For this review, take the finished solid that the model builds, in its own axes (mm). A direction names the side the tool comes from. Give positions to 0.01 mm unless a question says otherwise; leave off trailing zeros. Write each loop counter-clockwise with the first axis right and the second up, starting at its lowest first coordinate (ties: lowest second). Pieces come first, ordered by that corner, then holes.
1) For P1, Ø4, axis at x = -2, z = 25.5, coming from the -Y side; P2, Ø11, axis at y = -11, z = 47, coming from the -X side; P3, Ø3, axis at x = -0.5, y = 4.5, coming from the -Z side; P4, Ø3, axis at x = 0.5, z = 27.5, coming from the +Y side, all flat-tipped, find the tip position at first contact; note any pin that passes through.
2) Wall thickness on line 1 along Z through (x, y) = (-1.5, -16.5); line 2 along Y through (x, z) = (4, -2.5); line 3 along Y through (x, z) = (-0.75, 39): over which ranges is each line inside the solid? List them lowest first.
3) We need section C-C on x = 4. Give the boundary of the cut face in (y, z).
4) Draft analysis for pull direction Z (two halves, no side actions). For faces 4 (the face through (2, 15.24, 2)), 5 (the face through (2.451, 2.348, 10.305)), 6 (the face through (0.022, -0.354, 42.917)), 7 (the face through (0.54, 7.73, -2.44)), state which applies: pulls with the +Z half, pulls with the -Z half, needs draft (parallel to the pull), parting line crosses it, or undercut.
5) Machinability: for faces 1 (the face through (0, -17, 71.438)), 2 (the face through (-1.588, -1.5, 47.5)), 3 (the face through (0.07, 8.91, 8.89)), which of the approach directions +Z, -Z, +X, -X, +Y, -Y give a long, thin tool a straight path to every point of the face, cutting with its end or side? Answer none if there is none.
6) We need section D-D on z = 69. Give the boundary of the cut face in (x, y).
7) We need section A-A on z = 0. Give the boundary of the cut face in (x, y), and give its area (3 significant figures).
from build123d import *

# Parameters (mm, degrees)
F2_DEPTH      = 1.5875
F2_DEPTH_BACK = 1.5875
F3_DEPTH      = 9.525
F3_DEPTH_BACK = 9.525
F4_T1_DEPTH   = 62.865
F4_T6_DEPTH   = 62.865
F4_T11_DEPTH  = 62.865
F4_T16_DEPTH  = 62.865
F4_T21_DEPTH  = 62.865
F5_R          = 2.5
F6_DEPTH      = 34.1227081721
F7_R          = 1.3462
F8_DEPTH      = 25.4
F9_R          = 7.62
F10_R         = 0.635
F11_DEPTH     = 25.4
F12_R         = 1.27
F14_DEPTH     = 34.1227081721


# Not quite as in the source:
# - a fillet or chamfer that OpenCascade refuses, or shapes differently, is made with other operations: its cross-section is extruded or revolved along the edge and cut away or added
# - a feature names something its author has since deleted; it is built from what else it names


with BuildPart() as f2:
    # F1 (on Right) → F2 (new body, two sides)
    with BuildSketch(Plane.YZ) as f2_sk:
        with BuildLine():
            Line((-18.8817081721, 76.2), (-18.8817081721, 71.4375))
            Line((-18.8817081721, 71.4375), (-15.875, 71.4375))
            ThreePointArc((-15.875, 71.4375), (-14.541737999, 71.0594464463), (-13.6053613819, 70.0378247534))
            Line((-13.6053613819, 70.0378247534), (-1.35700712, 45.6593854024))
            ThreePointArc((-1.35700712, 45.6593854024), (-0.3438898526, 42.8769409358), (0, 39.9358282931))
            Line((0, 39.9358282931), (0, 8.89))
            Line((0, 8.89), (4.7625, 8.89))
            Line((4.7625, 8.89), (4.7625, 40.6322548497))
            ThreePointArc((4.7625, 40.6322548497), (4.4978433834, 42.8957264678), (3.7181513215, 45.0370875254))
            Line((3.7181513215, 45.0370875254), (-10.5324309359, 73.4006495068))
            ThreePointArc((-10.5324309359, 73.4006495068), (-12.4051841702, 75.4438928927), (-15.0717081721, 76.2))
            Line((-15.0717081721, 76.2), (-18.8817081721, 76.2))
        make_face()
    extrude(amount=F2_DEPTH)
    extrude(f2_sk.sketch, amount=-F2_DEPTH_BACK)

    # F1 (on Right) → F3 (join, two sides)
    with BuildSketch(Plane.YZ) as f3_sk:
        Polygon((4.7625, 8.89), (0, 8.89), (0, -8.89), (15.24, -8.89), (15.24, 8.89), align=None)
    extrude(amount=F3_DEPTH)
    extrude(f3_sk.sketch, amount=-F3_DEPTH_BACK)

    # F4: fillet of radius 9.525 on 4 edges, made by hand

    # F4_s2 → F4_t1 (cut)
    with BuildSketch(Plane.XZ.offset(-39.0525)):
        with BuildLine():
            ThreePointArc((9.525, 0.635), (6.7351920908, -6.1001920908), (0, -8.89))
            Line((0, -8.89), (9.525, -8.89))
            Line((9.525, -8.89), (9.525, 0.635))
        make_face()
        with BuildLine():
            ThreePointArc((-9.525, 0.635), (-6.7351920908, -6.1001920908), (0, -8.89))
            Line((0, -8.89), (-9.525, -8.89))
            Line((-9.525, -8.89), (-9.525, 0.635))
        make_face()
    extrude(amount=F4_T1_DEPTH, mode=Mode.SUBTRACT)


with BuildPart() as f4_tool4:
    # F4_s5 → F4_t6 (new body)
    with BuildSketch(Plane.XZ.offset(23.8125)):
        with BuildLine():
            ThreePointArc((0, 8.89), (6.7351920908, 6.1001920908), (9.525, -0.635))
            Line((9.525, -0.635), (9.525, 8.89))
            Line((9.525, 8.89), (0, 8.89))
        make_face()
    extrude(amount=-F4_T6_DEPTH)

    split(bisect_by=Plane.YZ.offset(1.5875), keep=Keep.TOP)


with BuildPart() as f2_1:
    add(f2.part)

    # F4_t3: cut F4_tool4
    add(f4_tool4.part, mode=Mode.SUBTRACT)


with BuildPart() as f4_tool9:
    # F4_s10 → F4_t11 (new body)
    with BuildSketch(Plane.XZ.offset(23.8125)):
        with BuildLine():
            ThreePointArc((0, 8.89), (6.7351920908, 6.1001920908), (9.525, -0.635))
            Line((9.525, -0.635), (9.525, 8.89))
            Line((9.525, 8.89), (0, 8.89))
        make_face()
    extrude(amount=-F4_T11_DEPTH)

    split(bisect_by=Plane.XZ.offset(-4.7625), keep=Keep.BOTTOM)


with BuildPart() as f2_2:
    add(f2_1.part)

    # F4_t8: cut F4_tool9
    add(f4_tool9.part, mode=Mode.SUBTRACT)


with BuildPart() as f4_tool14:
    # F4_s15 → F4_t16 (new body)
    with BuildSketch(Plane.XZ.offset(-39.0525)):
        with BuildLine():
            ThreePointArc((0, 8.89), (-6.7351920908, 6.1001920908), (-9.525, -0.635))
            Line((-9.525, -0.635), (-9.525, 8.89))
            Line((-9.525, 8.89), (0, 8.89))
        make_face()
    extrude(amount=F4_T16_DEPTH)

    split(bisect_by=Plane.XZ.offset(-4.7625), keep=Keep.BOTTOM)


with BuildPart() as f2_3:
    add(f2_2.part)

    # F4_t13: cut F4_tool14
    add(f4_tool14.part, mode=Mode.SUBTRACT)


with BuildPart() as f4_tool19:
    # F4_s20 → F4_t21 (new body)
    with BuildSketch(Plane.XZ.offset(-39.0525)):
        with BuildLine():
            ThreePointArc((0, 8.89), (-6.7351920908, 6.1001920908), (-9.525, -0.635))
            Line((-9.525, -0.635), (-9.525, 8.89))
            Line((-9.525, 8.89), (0, 8.89))
        make_face()
    extrude(amount=F4_T21_DEPTH)

    split(bisect_by=Plane.YZ.offset(-1.5875), keep=Keep.BOTTOM)


with BuildPart() as f2_4:
    add(f2_3.part)

    # F4_t18: cut F4_tool19
    add(f4_tool19.part, mode=Mode.SUBTRACT)

    # F5 (on face) → F6 (cut, through all)
    with BuildSketch(Plane(origin=(0, 15.24, 0), x_dir=(-1, 0, 0), z_dir=(0, 1, 0))):
        Circle(F5_R)
    extrude(amount=-F6_DEPTH, mode=Mode.SUBTRACT)

    # F7 (on Top) → F8 (cut)
    with BuildSketch(Plane.XY):
        with Locations((0, 10.5804353952)):
            Circle(F7_R)
        with Locations((0, -26.9685275853)):
            Circle(F7_R)
    extrude(amount=F8_DEPTH, mode=Mode.SUBTRACT)

    # F9
    f9_edges = [f2_4.edges().sort_by_distance(p)[0] for p in [
        (-9.50381, 7.62, 0),
        (-1.5875, 2.38125, 8.756777),
        (1.5875, 2.38125, 8.756777),
    ]]
    fillet(f9_edges, radius=F9_R)

    # F10 (on face) → F11 (cut)
    with BuildSketch(Plane.XY.offset(76.2)):
        with Locations((0, -15.8845081721)):
            Circle(F10_R)
    extrude(amount=-F11_DEPTH, mode=Mode.SUBTRACT)

    # F12
    f12_edges = [f2_4.edges().sort_by_distance(p)[0] for p in [
        (1.5875, -18.881708, 73.81875),
        (-1.5875, -18.881708, 73.81875),
    ]]
    fillet(f12_edges, radius=F12_R)

    # F13 (on face) → F14 (cut, through all)
    with BuildSketch(Plane(origin=(0, 15.24, 0), x_dir=(-1, 0, 0), z_dir=(0, 1, 0))):
        Polygon((-4.7625, -11.6415646072), (-4.7625, 10.8039603039), (-9.6872693895, 10.8039603039), (-9.6872693895, -15.5402623288), (11.7396748797, -15.5402623288), (11.7396748797, 10.8039603039), (4.7625, 10.8039603039), (4.7625, -11.6415646072), align=None)
    extrude(amount=-F14_DEPTH, mode=Mode.SUBTRACT)


solid = f2_4.part
Results list:
1. P1: stops at y = 0
1. P2: passes through
1. P3: stops at z = -8.89
1. P4: stops at y = 4.76
2. line 1: z = 71.44 to 76.2
2. line 2: y = 0 to 15.24
2. line 3: y = 0 to 4.76
3. outline: (0, -8.01) - (15.24, -8.01) - (15.24, 8.01) - (4.76, 8.01) - (4.76, 8.26) - (0, 8.26) - close
4. face 4: needs draft
4. face 5: pulls with the +Z half
4. face 6: pulls with the -Z half
4. face 7: undercut
5. face 1: -Z, +X, -X, -Y
5. face 2: +Z, -X, +Y, -Y
5. face 3: +Z, +Y
6. outline: (-1.59, -13.08) - (1.59, -13.08) - (1.59, -8.32) - (-1.59, -8.32) - close
7. outline: (-4.76, 0) - (-2.5, 0) - (-2.5, 15.24) - (-4.76, 15.24) - close; (2.5, 0) - (4.76, 0) - (4.76, 15.24) - (2.5, 15.24) - close
7. area: 69.0 mm2
